The listing builds one solid part. Answer for the finished solid, in the listing's coordinates (mm). Face numbers are marked on the shaded views. Coordinates: 2 decimals unless noted, no trailing zeros. Write each loop counter-clockwise with the first axis right and the second up, starting at its lowest first coordinate (ties: lowest second). Pieces come first, ordered by that corner, then holes.
from build123d import *

# Parameters (mm, degrees)
SKETCH_1_R          = 1.5
SKETCH_1_R_2        = 1.5000000000000007
EXTRUDE_1_DEPTH     = 3
EXTRUDE_2_DEPTH     = 3
EXTRUDE_3_DEPTH     = 10
EXTRUDE_4_DEPTH     = 3
SKETCH_5_W          = 5.158542288566252
SKETCH_5_H          = 3
EXTRUDE_5_DEPTH     = 2
SKETCH_6_W          = 7
SKETCH_6_H          = 3
EXTRUDE_6_DEPTH     = 2
CHAMFER_1_SIZE      = 3
SKETCH_7_W          = 66.6001387822102
SKETCH_7_H          = 28.97194366122671
CUT_EXTRUDE_1_DEPTH = 80
EXTRUDE_8_DEPTH     = 3
SKETCH_10_R         = 1.4999999999999987
SKETCH_10_R_2       = 1.5000000000000007
CUT_EXTRUDE_2_DEPTH = 3


with BuildPart() as part:
    # 草图1 → 凸台-拉伸1 (new body)
    with BuildSketch(Plane(origin=(0, 0, 0), x_dir=(1, 0, 0), z_dir=(0, 1, 0))):
        with BuildLine():
            Line((0, 2.999999999999999), (25, 2.999999999999999))
            ThreePointArc((25, 2.999999999999999), (28, 0), (25, -2.999999999999999))
            Line((25, -2.999999999999999), (0, -2.999999999999999))
            ThreePointArc((0, -2.999999999999999), (-2.999999999999997, 3.7e-16), (0, 2.999999999999999))
        make_face()
        with Locations(Location((0, 0, 0), (0, 0, 270))):
            Circle(SKETCH_1_R, mode=Mode.SUBTRACT)
        with Locations(Location((25, 0, 0), (0, 0, 270))):
            Circle(SKETCH_1_R_2, mode=Mode.SUBTRACT)
    extrude(amount=EXTRUDE_1_DEPTH)

    # 草图2 → 凸台-拉伸2 (add)
    with BuildSketch(Plane.XZ):
        with BuildLine():
            Line((26.499999999999986, -2.5980762113533244), (46.006930637676454, 8.664255443372392))
            Line((46.006930637676454, 8.664255443372392), (56.006930637676454, 8.664255443372392))
            Line((56.006930637676454, 8.664255443372392), (56.00693063767646, 9.66425544337239))
            Line((56.00693063767646, 9.66425544337239), (46.006930637676476, 9.66425544337241))
            Line((46.006930637676476, 9.66425544337241), (26.942439211337344, 2.7051474006582077))
            Line((26.942439211337344, 2.7051474006582077), (25.518180954342487, 2.9549092200195775))
            ThreePointArc((25.518180954342487, 2.9549092200195775), (27.954179309279922, 0.522326151578114), (26.499999999999986, -2.5980762113533244))
        make_face()
    extrude(amount=-EXTRUDE_2_DEPTH)

    # 草图3 → 凸台-拉伸3 (add)
    with BuildSketch(Plane(origin=(56.0069306376764, 0, -3.8863e-13), x_dir=(-6.94e-15, 0, -1), z_dir=(1, 0, -6.94e-15))):
        with BuildLine():
            Line((-14.664255443372781, 16), (-14.664255443372781, 14.245195173083879))
            ThreePointArc((-14.664255443372781, 14.245195173083879), (-9.864255443372706, 1.5000000000000009), (-14.664255443372777, -11.24519517308388))
            Line((-14.664255443372777, -11.24519517308388), (-14.664255443372777, -13))
            ThreePointArc((-14.664255443372777, -13), (-8.66425544337271, 1.5000000000000009), (-14.664255443372781, 16))
        make_face()
    extrude(amount=-EXTRUDE_3_DEPTH)

    # 草图4 → 凸台-拉伸4 (add)
    with BuildSketch(Plane(origin=(0, 3, 0), x_dir=(1, 0, 0), z_dir=(0, 1, 0))):
        Polygon((38.75296926264814, -4.476178890808707), (51.00693063767646, -8.719151204865875), (46.006930637676454, -8.664255443372392), align=None)
    extrude(amount=-EXTRUDE_4_DEPTH)

    # 草图5 → 凸台-拉伸5 (add)
    with BuildSketch(Plane(origin=(0, 0, 8.664255443372392), x_dir=(-1, 0, 0), z_dir=(0, 0, -1))):
        with Locations((-53.42765949339333, 1.5)):
            Rectangle(SKETCH_5_W, SKETCH_5_H)
    extrude(amount=EXTRUDE_5_DEPTH)

    # 草图6 → 凸台-拉伸6 (add)
    with BuildSketch(Plane(origin=(0, 0, 6.664255443372392), x_dir=(-1, 0, 0), z_dir=(0, 0, -1))):
        with Locations((-47.3483883491102, 1.5)):
            Rectangle(SKETCH_6_W, SKETCH_6_H)
    extrude(amount=-EXTRUDE_6_DEPTH)

    # 倒角1
    chamfer_1_edges = [part.edges().sort_by_distance(p)[0] for p in [
        (56.006930637676454, 1.5, 6.664255443372392),
    ]]
    chamfer(chamfer_1_edges, length=CHAMFER_1_SIZE)

    # 草图7 → 切除-拉伸1 (cut)
    with BuildSketch(Plane.XZ):
        with Locations((-6.222464944833996, 7.620791926380881)):
            Rectangle(SKETCH_7_W, SKETCH_7_H)
    extrude(amount=-CUT_EXTRUDE_1_DEPTH, mode=Mode.SUBTRACT)

    # 草图8 → 凸台-拉伸8 (add)
    with BuildSketch(Plane.XZ):
        with BuildLine():
            Line((29.005967275330715, -2.053188022146578), (11.386945083594192, -16.83730304493695))
            ThreePointArc((11.386945083594192, -16.83730304493695), (7.160448925177645, -16.46753254463963), (7.530219425474969, -12.241036386223078))
            Line((7.530219425474969, -12.241036386223078), (25.14924161721149, 2.5430786365672917))
            ThreePointArc((25.14924161721149, 2.5430786365672917), (29.37573777562804, 2.173308136269972), (29.005967275330715, -2.053188022146578))
        make_face()
    extrude(amount=-EXTRUDE_8_DEPTH)

    # 草图10 → 切除-拉伸2 (cut)
    with BuildSketch(Plane(origin=(0, 3, 0), x_dir=(1, 0, 0), z_dir=(0, 1, 0))):
        with Locations(Location((9.458582254534583, 14.539169715580016, 0), (0, 0, 270))):
            Circle(SKETCH_10_R)
        with Locations(Location((27.077604446271103, -0.24494530721035945, 0), (0, 0, 270))):
            Circle(SKETCH_10_R_2)
    extrude(amount=-CUT_EXTRUDE_2_DEPTH, mode=Mode.SUBTRACT)


solid = part.part
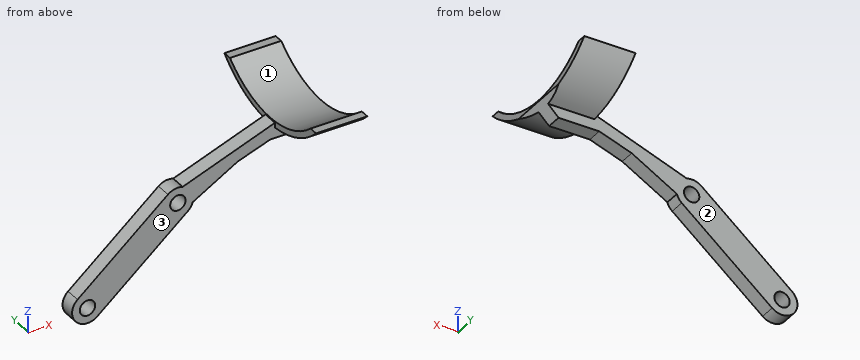
Q1. The part is cut by section C-C, the plane z = -10. Write down the section's boundary in (x, y), then the cut area to 3 significant figures.
Answers below:
outline: (10.2, 0) - (19.54, 0) - (19.54, 3) - (10.2, 3) - close
area: 28.0 mm2
Q2. Determine the mould class of the marked faces 1, 2 and 3 for opening direction Y: released by +Y, released by -Y, zero draft, split by the parting line, or undercut.
Answers below:
face 1: undercut
face 2: released by +Y
face 3: released by -Y
Q3. The part is cut by section A-A, the plane z = 0.5. Write down the section's boundary in (x, y), then the cut area to 3 significant figures.
Answers below:
outline: (22.71, 0) - (25.6, 0) - (25.6, 3) - (22.71, 3) - close; (28.56, 0) - (31.87, 0) - (31.87, 3) - (28.56, 3) - close
area: 18.6 mm2
Q4. Find the intervals of material crossed by probe 1 along Y at (x, z) = (46.5, 8); probe 2 along Z at (x, y) = (51.5, -1.25); probe 3 along Z at (x, y) = (21.5, 1.25), in increasing order.
Answers below:
probe 1: y = 0 to 3
probe 2: z = 8.85 to 10.06
probe 3: z = -8.35 to -0.52
Q5. The part is cut by section B-B, the plane y = 9.5. Write down the section's boundary in (x, z), then the cut area to 3 significant figures.
Answers below:
outline: (46.01, 10.29) - (56.01, 10.29) - (56.01, 11.6) - (46.01, 11.6) - close
area: 13.1 mm2
Q6. Given pin 1 (10 mm diameter, centred on x = 39.5, y = 0, fed in from -Z); pin 2 (12 mm diameter, centred on x = 38, z = 10.5, fed in from -Y); pin 3 (1.5 mm diameter, centred on x = 50, y = 2, fed in from -Z), each flat-ended and moving along its own axis, determine where each tip first touches the part or whether it passes through.
Answers below:
pin 1: stops at z = 2.02
pin 2: stops at y = 0
pin 3: stops at z = 6.66
